Source: three-view drawing plus pictorial views. Frame: mm from the lowest corner of the part. Give positions to 0.01 mm unless a question says otherwise; leave off trailing zeros. Order: outer loops, then holes, each group sorted by start corner. A loop starts at its lowest first (then second) coordinate and runs counter-clockwise, first axis right, second up.
1) Section A-A, the plane x = 7. Return loops of the section in (y, z) (1 decimal), plus the area to 3 significant figures.
2) Section C-C, the plane x = 100. Return loops of the section in (y, z) (1 decimal).
3) Material intervals for line 1 (Y direction, x = 6, z = 0.25); line 2 (Y direction, x = 86, z = 2.45); line 3 (X direction, y = 33.5, z = 1.35), sorted ascending.
4) Section D-D, the plane z = 0.9. Give the number of separate pieces and of enclosed holes in the cut face, plus the area to 3 significant figures.
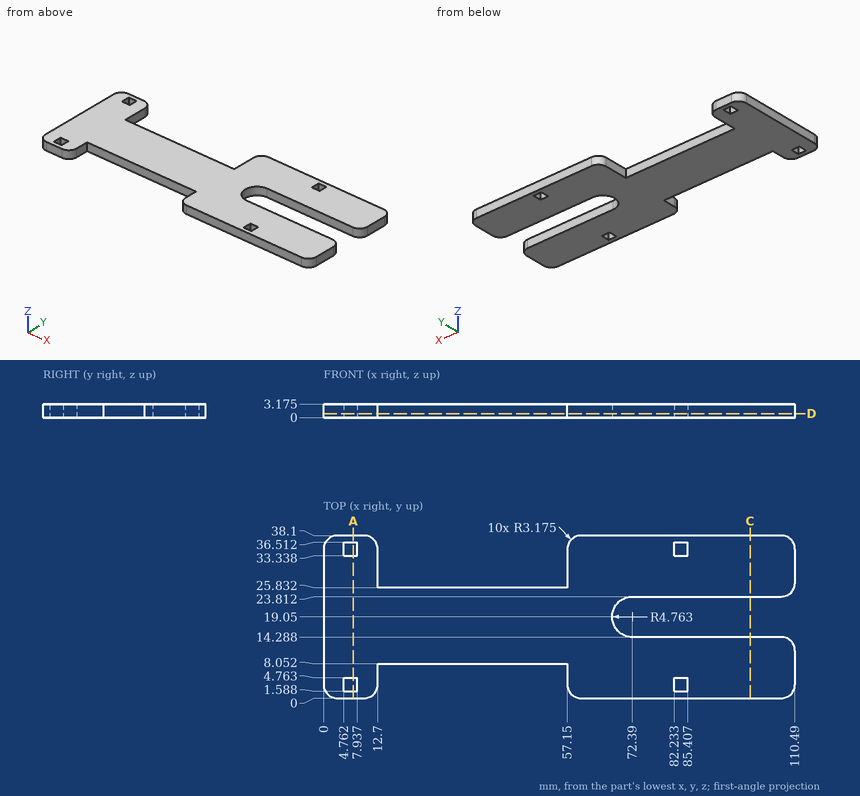
From the geometry:
1. outline: (0, 0) - (1.6, 0) - (1.6, 3.2) - (0, 3.2) - close; (4.8, 0) - (33.3, 0) - (33.3, 3.2) - (4.8, 3.2) - close; (36.5, 0) - (38.1, 0) - (38.1, 3.2) - (36.5, 3.2) - close
1. area: 101 mm2
2. outline: (0, 0) - (14.3, 0) - (14.3, 3.2) - (0, 3.2) - close; (23.8, 0) - (38.1, 0) - (38.1, 3.2) - (23.8, 3.2) - close
3. line 1: y = 0 to 1.59, 4.76 to 33.34, 36.51 to 38.1
3. line 2: y = 0 to 14.29, 23.81 to 38.1
3. line 3: x = 0 to 4.76, 7.94 to 12.7, 57.15 to 82.23, 85.41 to 110.49
4. separate pieces: 1
4. enclosed holes: 4
4. area: 2,850 mm2
